Could you check a few things on this model? Use its own coordinates, in mm. A direction names the side the tool comes from. Round coordinates to 2 decimals unless told otherwise and drop trailing zeros. Loops run counter-clockwise (first coordinate to the right, second up) from the corner with the lowest first, then second, coordinate; pieces in that order, holes last. Notation, with made-up numbers: (-17.5, -22.75) - (-10.5, -22.75) arc R22 ccw to (-10.5, 6.25) - close; hole circle Ø1 at (72.25, 6). An arc over 180 degrees is marked (long way). Put each result on its own line as item: value. Start each with the question number.
from build123d import *

# Parameters (mm, degrees)
F1_DEPTH = 3.5
F2_W     = 3.5
F2_H     = 10
F3_DEPTH = 3.5


with BuildPart() as f1:
    # F0 (on Top) → F1 (new body)
    with BuildSketch(Plane.XY):
        Polygon((63.617211, -14), (63.617211, 0), (63.617211, 6.802419), (34.359907, 13.436434), (35.133875, 16.849786), (25.38144, 19.061125), (24.607472, 15.647772), (-24.37305, 26.753974), (-23.599082, 30.167326), (-33.351517, 32.378664), (-34.125485, 28.965312), (-63.382789, 35.599327), (-63.382789, 0), (-66.882789, 0), (-66.882789, -14), (-63.382789, -12), (-63.382789, -22), (-66.882789, -20), (-66.882789, -40), (-63.382789, -38), (-63.382789, -48), (-66.882789, -46), (-66.882789, -60), (-63.382789, -60), (60.117211, -60), (63.617211, -60), (63.617211, -46), (60.117211, -48), (60.117211, -38), (63.617211, -40), (63.617211, -20), (60.117211, -22), (60.117211, -12), align=None)
    extrude(amount=F1_DEPTH)

    # F2 (on face) → F3 (cut)
    with BuildSketch(Plane.XY.offset(3.5)):
        with Locations((14.367211, -15)):
            Rectangle(F2_W, F2_H)
        with Locations((14.367211, -45)):
            Rectangle(F2_W, F2_H)
    extrude(amount=-F3_DEPTH, mode=Mode.SUBTRACT)


solid = f1.part
Item 1: Thinking about a two-plate mould opening in Y: for faces 1 (the face through (-3, -22, 3.5)), 2 (the face through (61.843, -38.986, 1.726)), 3 (the face through (-33.733, 30.696, 1.726)), 4 (the face through (-3, -60, 2)), which applies, released by +Y, released by -Y, zero draft, split by the parting line, or undercut?
Item 2: I need wall thicknesses on line 1 (Y direction, x = 14, z = 0.3); line 2 (X direction, y = -13.5, z = 0.8); line 3 (X direction, y = 5.5, z = 0.2). Which ranges of each line are inside material? Lowest first, please. Write a range as from..to.
Item 3: On a 3-axis mill with a long thin cutter (end or side, diameter ignored), from which of +Z, -Z, +X, -X, +Y, -Y can I reach the whole of each face in a straight line? I mean faces 5 (the face through (34.74, 15.12, 1.73)), 6 (the face through (-65, 0, 2)), 7 (the face through (14, -40, 2)). Say none if no direction works.
Item 4: Will these pins go through, and if not, where does the flat tip stop? P1, Ø1.8, axis at y = -42.5, z = 2, coming from the -X side; P2, Ø1, axis at x = 14, z = 1, coming from the +Y side; P3, Ø1.7, axis at x = 15, z = 1.5, coming from the +Y side.
Item 5: Suppose I cut it at B-B, the plane x = -43.5. List the corners of the cut face in (y, z) for me.
Item 6: Suppose I cut it at A-A, the plane z = 1.9. Count the separate pieces of the cut face and the enclosed holes in it, then the cut area to 3 significant figures.
Item 7: Suppose I cut it at C-C, the plane x = 6.5. List the corners of the cut face in (y, z) for me.
Numbers:
1. face 1: zero draft
1. face 2: undercut
1. face 3: released by +Y
1. face 4: released by -Y
2. line 1: -60..-50, -40..-20, -10..18.05
2. line 2: -66.88..-66.01, -63.38..12.62, 16.12..60.12, 62.74..63.62
2. line 3: -63.38..63.62
3. face 5: +Z, -Z, +X
3. face 6: +Z, -Z, -X, +Y
3. face 7: +Z, -Z
4. P1: x = -63.38
4. P2: y = 18.17
4. P3: y = 18.02
5. outline: (-60, 0) - (31.09, 0) - (31.09, 3.5) - (-60, 3.5) - close
6. separate pieces: 1
6. enclosed holes: 2
6. area: 10,400 mm^2
7. outline: (-60, 0) - (19.75, 0) - (19.75, 3.5) - (-60, 3.5) - close
